```python
from build123d import *

# Parameters (mm, degrees)
SKETCH1_R           = 1.5875
BOSS_EXTRUDE1_DEPTH = 0.79375


with BuildPart() as part:
    # Sketch1 → Boss-Extrude1 (new, symmetric)
    with BuildSketch(Plane(origin=(0, 0, 0), x_dir=(1, 0, 0), z_dir=(0, 1, 0))):
        with BuildLine():
            ThreePointArc((-21.319139699, 4.975774091), (0, -1.536759472), (21.319139699, 4.975774091))
            ThreePointArc((21.319139699, 4.975774091), (29.647774091, 3.352860301), (28.024860301, -4.975774091))
            ThreePointArc((28.024860301, -4.975774091), (0, -13.536759472), (-28.024860301, -4.975774091))
            ThreePointArc((-28.024860301, -4.975774091), (-29.647774091, 3.352860301), (-21.319139699, 4.975774091))
        make_face()
        with Locations(Location((-24.672, 0, 0), (0, 0, 270))):
            Circle(SKETCH1_R, mode=Mode.SUBTRACT)
        with Locations(Location((24.672, 0, 0), (0, 0, 270))):
            Circle(SKETCH1_R, mode=Mode.SUBTRACT)
    extrude(amount=BOSS_EXTRUDE1_DEPTH, both=True)


solid = part.part
```
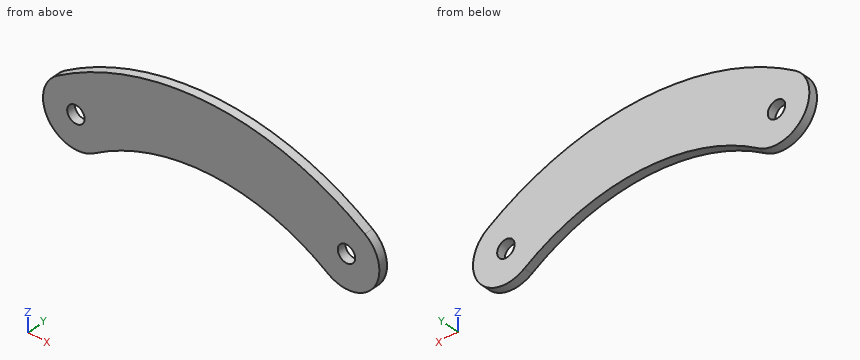
The listing builds one solid part. Answer for the finished solid, in the listing's coordinates (mm). Coordinates: 2 decimals unless noted, no trailing zeros. Loops run counter-clockwise (first coordinate to the right, second up) from the corner with the lowest first, then second, coordinate; pieces in that order, holes last. Notation, with made-up numbers: M -21.5,33.25 L 12.5,33.25 A25 ccw 12.5,45.25 Z; hole C 6.25,-14 d4. An arc over 180 degrees is marked long. Answer as CSV lines item,"result". Start each with the question number.
(1) The part is cut by section D-D (x = -4.5). Give the vertices of the cut face in (y, z), and give its area (3 significant figures).
(2) The part is cut by section B-B (y = 0.05). Give the vertices of the cut face in (x, z) (1 decimal), and give its area (3 significant figures).
(3) Find the intervals of material crossed by L1, parallel to Z at x = 24.5, y = 0; L2, parallel to Z at x = -25, y = 0; L3, parallel to X at y = 0.7, z = -4.5, in increasing order. Write a range as [from, to].
(4) Given pin 1 (3 mm diameter, centred on x = 24.672, z = 0, fed in from -Y), flat-ended and moving along its own axis, determine where the tip first touches the part or whether it passes through.
(5) The part is cut by section A-A (z = 0). Give the vertices of the cut face in (x, y).
(6) The part is cut by section C-C (z = -2.5). Give the vertices of the cut face in (x, y), and give its area (3 significant figures).
Determined:
1,outline,"M -0.79,1.27 L 0.79,1.27 L 0.79,13.33 L -0.79,13.33 Z"
1,area,"19.2 mm2"
2,outline,"M -28,5 A6 ccw -21.3,-5 A38.2 cw 21.3,-5 A6 ccw 28,5 A50.2 ccw Z; hole C -24.7,0 d3.2; hole C 24.7,0 d3.2"
2,area,"726 mm2"
3,L1,"[-6, -1.58], [1.58, 7.15]"
3,L2,"[-5.99, -1.55], [1.55, 6.86]"
3,L3,"[-28.64, -20.6], [20.6, 28.64]"
4,pin 1,"through"
5,outline,"M -30.67,-0.79 L -26.26,-0.79 L -26.26,0.79 L -30.67,0.79 Z; M -23.08,-0.79 L -10.72,-0.79 L -10.72,0.79 L -23.08,0.79 Z; M 10.72,-0.79 L 23.08,-0.79 L 23.08,0.79 L 10.72,0.79 Z; M 26.26,-0.79 L 30.67,-0.79 L 30.67,0.79 L 26.26,0.79 Z"
6,outline,"M -30.13,-0.79 L -17.08,-0.79 L -17.08,0.79 L -30.13,0.79 Z; M 17.08,-0.79 L 30.13,-0.79 L 30.13,0.79 L 17.08,0.79 Z"
6,area,"41.4 mm2"
